Geometry: final body of the model. Coordinates: model frame, mm. A direction names the side the tool comes from. Round coordinates to 2 decimals unless told otherwise and drop trailing zeros. Write each loop counter-clockwise with the first axis right and the second up, starting at its lowest first coordinate (ties: lowest second). Pieces come first, ordered by that corner, then holes. Notation, with made-up numbers: (59.25, 75.5) - (104.25, 75.5) arc R21 ccw to (104.25, 106.5) - close; hole circle Ø3 at (87.5, -29). An arc over 180 degrees is marked (long way). Write each question's results on one line, items separated by ' | '.
Solid Edge part; units mm, degrees
sketch "Sketch1" plane through (0, 0, 0) normal (0, 0, 1) x (1, 0, 0)
  line L0 (-25, -12.5) -> (25, -12.5)
  line L1 (25, -12.5) -> (25, 12.5)
  line L2 (25, 12.5) -> (-25, 12.5)
  line L3 (-25, 12.5) -> (-25, -12.5)
extrude "Protrusion1" add sketch "Sketch1" along normal blind 3
sketch "Sketch2" plane through (0, -12.5, 1.5) normal (0, -1, 0) x (1, 0, 0)
  line L0 (-1.1982, 0.5492) -> (1.1982, 0.5492)
  line L1 (1.1982, 0.5492) -> (1.1982, 2.4508)
  line L2 (1.1982, 2.4508) -> (-1.1982, 2.4508)
  line L3 (-1.1982, 2.4508) -> (-1.1982, 0.5492)
extrude "Kivágás_1" cut sketch "Sketch2" against normal blind 36.6689 and the other way blind 13.795
Q1. Ray query, line 1 along Z through (x, y) = (0.5, -8.25). Return the intervals inside material, ascending.
Answer block:
line 1: 0 to 2.05
Q2. Section query B-B, the plane y = 6.75. Return loops of the section in (x, z), plus the area to 3 significant figures.
Answer block:
outline: (-25, 0) - (25, 0) - (25, 3) - (1.2, 3) - (1.2, 2.05) - (-1.2, 2.05) - (-1.2, 3) - (-25, 3) - close | area: 148 mm2
Q3. Access query for faces 1 (the flat face through (1.198, -0.2, 2.5)), 2 (the flat face through (0, 0, 0)). Directions: +Z, -Z, +X, -X, +Y, -Y. A direction counts if a zero-diameter tool reaches every point of the face in a straight line with its end or side. Return the directions, or none.
Answer block:
face 1: +Z, +Y, -Y | face 2: -Z, +X, -X, +Y, -Y
Q4. Section query A-A, the plane z = 2.55. Return loops of the section in (x, y).
Answer block:
outline: (-25, -12.5) - (-1.2, -12.5) - (-1.2, 12.5) - (-25, 12.5) - close; (1.2, -12.5) - (25, -12.5) - (25, 12.5) - (1.2, 12.5) - close
Q5. Pin query (flat end, axial travel): pin 1 (2.5 mm diameter, centred on x = 0, y = 2, fed in from +Z). Return the tip coordinate at first contact, or that it passes through.
Answer block:
pin 1: z = 3
Q6. Mould query, pull axis X, two halves, no side actions, for faces 3 (the flat face through (0, -12.5, 1)), 4 (the flat face through (-25, 0, 1)), 5 (the flat face through (-1.198, -0.2, 2.5)). Classes: pulls with the +X half, pulls with the -X half, needs draft (parallel to the pull), parting line crosses it, or undercut.
Answer block:
face 3: needs draft | face 4: pulls with the -X half | face 5: undercut
